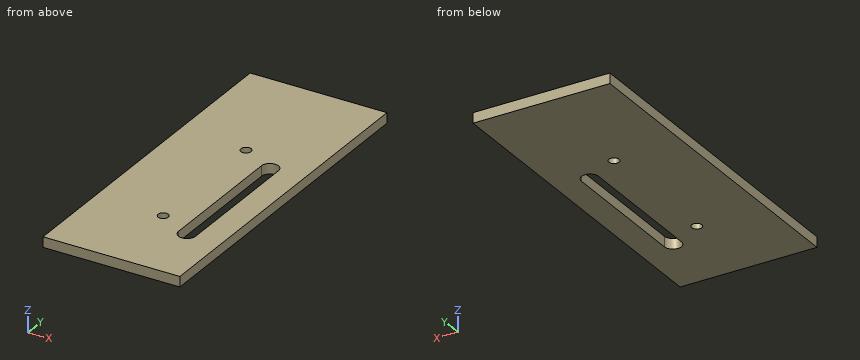
```python
from build123d import *

# Parameters (mm, degrees)
F1_DEPTH = 3
F3_D     = 3
F6_DEPTH = 25


with BuildPart() as f1:
    # F0 (on Top) → F1 (new body)
    with BuildSketch(Plane.XY):
        Polygon((0, 100), (0, 0), (5.765755, 0), (40, 0), (40, 100), align=None)
    extrude(amount=F1_DEPTH)

    # F3 (through all)
    with Locations(Plane.XY.offset(3)):
        with Locations((20, 65), (20, 25)):
            Hole(F3_D / 2)

    # F5 (on face) → F6 (cut)
    with BuildSketch(Plane.XY.offset(3)):
        with BuildLine():
            ThreePointArc((27.5, 20), (30, 17.5), (32.5, 20))
            Line((32.5, 20), (32.5, 60))
            ThreePointArc((32.5, 60), (30, 62.5), (27.5, 60))
            Line((27.5, 60), (27.5, 20))
        make_face()
    extrude(amount=-F6_DEPTH, mode=Mode.SUBTRACT)


solid = f1.part
```
Design review of the part built by this model. Coordinates are the model's own, in mm. Coordinates: 2 decimals unless noted, no trailing zeros. Write each loop counter-clockwise with the first axis right and the second up, starting at its lowest first coordinate (ties: lowest second). Pieces come first, ordered by that corner, then holes. Notation, with made-up numbers: M 88.25,4.5 L 124.25,4.5 A19 ccw 124.25,26.5 Z; hole C -36,-28.5 d4. An arc over 180 degrees is marked long. Answer as a JSON object with one key per item and string values.
Item 1: Add section B-B, the plane y = 25. Give the boundary of the cut face in (x, z).
Outcome:
{"outline": "M 0,0 L 18.5,0 L 18.5,3 L 0,3 Z; M 21.5,0 L 27.5,0 L 27.5,3 L 21.5,3 Z; M 32.5,0 L 40,0 L 40,3 L 32.5,3 Z"}
Item 2: Add section C-C, the plane z = 0.7. Give the boundary of the cut face in (x, y).
Outcome:
{"outline": "M 0,0 L 40,0 L 40,100 L 0,100 Z; hole C 20,25 d3; hole C 20,65 d3; hole M 27.5,20 A2.5 ccw 32.5,20 L 32.5,60 A2.5 ccw 27.5,60 Z"}
Item 3: Add section D-D, the plane y = 36. Give the boundary of the cut face in (x, z), and give its area (3 significant figures).
Outcome:
{"outline": "M 0,0 L 27.5,0 L 27.5,3 L 0,3 Z; M 32.5,0 L 40,0 L 40,3 L 32.5,3 Z", "area": "105 mm²"}
Item 4: Wall thickness on probe 1 along Y at (x, z) = (20, 0.7); probe 2 along X at (y, z) = (65, 2); probe 3 along X at (y, z) = (40, 0.95): over which ranges is each line inside the solid? List them lowest first.
Outcome:
{"probe 1": "0 to 23.5, 26.5 to 63.5, 66.5 to 100", "probe 2": "0 to 18.5, 21.5 to 40", "probe 3": "0 to 27.5, 32.5 to 40"}
Item 5: Add section A-A, the plane x = 30. Give the boundary of the cut face in (y, z).
Outcome:
{"outline": "M 0,0 L 17.5,0 L 17.5,3 L 0,3 Z; M 62.5,0 L 100,0 L 100,3 L 62.5,3 Z"}
